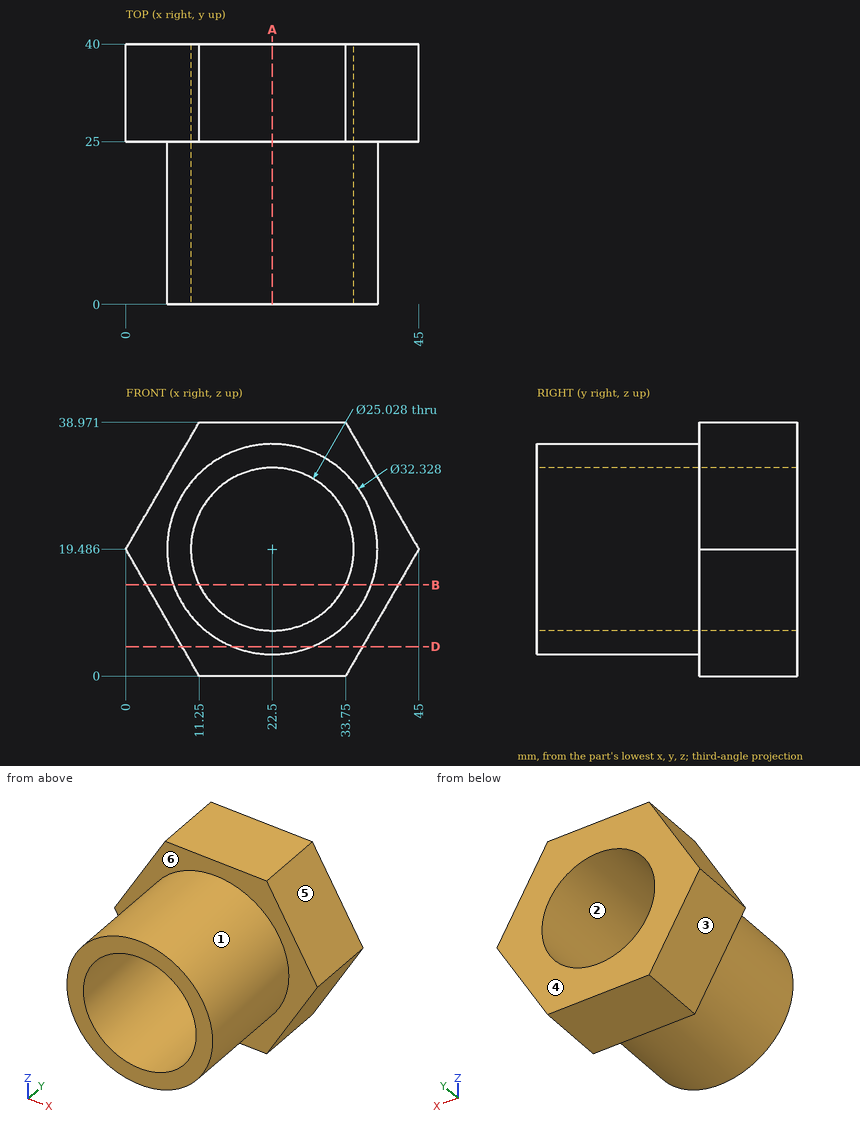
Study the drawing (mm; zero at the part's minimum x, y, z) and answer. A direction names the side the tool comes from. Coordinates: 2 decimals unless noted, no trailing zeros. Write each loop counter-clockwise with the first axis right and the second up, starting at its lowest first coordinate (ties: lowest second). Pieces come first, ordered by that corner, then holes. Notation, with made-up numbers: M 45,35.25 L 68,35.25 A29 cw 68,70.25 Z; hole C 36,65.25 d2. An arc over 180 degrees is marked long. Use a Markdown table: item, result. Add a question column.
1. Section D-D (z = 4.5) is taken. Give the vertices of the cut face in (x, y).
2. Section B-B (z = 14) is taken. Give the vertices of the cut face in (x, y) (1 decimal).
3. Which of the six approach directions +Z, -Z, +X, -X, +Y, -Y give full straight-line access (tool end or side, diameter ignored) to the marked faces 5 and 6?
4. Given P1, Ø6, axis at y = 10, z = 18, coming from the +X side; P2, Ø3, axis at x = 13.5, y = 16.5, coming from the +Z side (1 decimal); P3, Ø4, axis at y = 34, z = 23.5, coming from the +X side, each flat-ended and moving along its own axis, determine where each tip first touches the part or whether it passes through.
5. Section A-A (x = 22.5) is taken. Give the vertices of the cut face in (y, z).
6. Straight lines are drawn through the part: line 1 along Z through (x, y) = (22.5, 23.5); line 2 along Z through (x, y) = (22.5, 30); line 3 along Y through (x, z) = (34, 36). For each, find the intervals that lie inside material, in ascending order. Write a range as [from, to].
7. For a pull along X with two mould halves and no side action, classify the marked faces 1, 2, 3 and 4 as +X half, -X half, draft (parallel to the pull), parting line (faces both ways), or undercut.
Data:
| question | item | result |
|---|---|---|
| 1 | outline | M 8.65,25 L 16.44,25 L 16.44,0 L 28.56,0 L 28.56,25 L 36.35,25 L 36.35,40 L 8.65,40 Z |
| 2 | outline | M 3.2,25 L 7.3,25 L 7.3,0 L 11.3,0 L 11.3,40 L 3.2,40 Z; M 33.7,0 L 37.7,0 L 37.7,25 L 41.8,25 L 41.8,40 L 33.7,40 Z |
| 3 | face 5 | +Z, +X, +Y, -Y |
| 3 | face 6 | -Y |
| 4 | P1 | stops at x = 38.66 |
| 4 | P2 | stops at z = 33.8 |
| 4 | P3 | stops at x = 43.84 |
| 5 | outline | M 0,3.32 L 25,3.32 L 25,0 L 40,0 L 40,6.97 L 0,6.97 Z; M 0,32 L 40,32 L 40,38.97 L 25,38.97 L 25,35.65 L 0,35.65 Z |
| 6 | line 1 | z = [3.32, 6.97], [32, 35.65] |
| 6 | line 2 | z = [0, 6.97], [32, 38.97] |
| 6 | line 3 | y = [25, 40] |
| 7 | face 1 | parting line |
| 7 | face 2 | undercut |
| 7 | face 3 | -X half |
| 7 | face 4 | draft |
